from build123d import *

# Parameters (mm, degrees)
F0_R     = 3.302
F1_DEPTH = 6.35


with BuildPart() as f1:
    # F0 (on Top) → F1 (new body)
    with BuildSketch(Plane.XY):
        with BuildLine():
            ThreePointArc((12.671918, -0.844097), (12.692977, -0.422282), (12.7, 0))
            ThreePointArc((12.7, 0), (12.692977, 0.422282), (12.671918, 0.844097))
            ThreePointArc((12.671918, 0.844097), (12.507058, 2.205332), (12.196406, 3.540859))
            ThreePointArc((12.196406, 3.540859), (11.934096, 4.343656), (11.619009, 5.127243))
            ThreePointArc((11.619009, 5.127243), (10.998523, 6.35), (10.249828, 7.498736))
            ThreePointArc((10.249828, 7.498736), (9.728764, 8.163403), (9.164677, 8.791968))
            ThreePointArc((9.164677, 8.791968), (8.163403, 9.728764), (7.066969, 10.552154))
            ThreePointArc((7.066969, 10.552154), (6.35, 10.998523), (5.604949, 11.396251))
            ThreePointArc((5.604949, 11.396251), (4.343656, 11.934096), (3.031729, 12.332827))
            ThreePointArc((3.031729, 12.332827), (2.205332, 12.507058), (1.369182, 12.625979))
            ThreePointArc((1.369182, 12.625979), (0.685591, 12.681481), (0, 12.7))
            ThreePointArc((0, 12.7), (-0.685591, 12.681481), (-1.369182, 12.625979))
            ThreePointArc((-1.369182, 12.625979), (-2.205332, 12.507058), (-3.031729, 12.332827))
            ThreePointArc((-3.031729, 12.332827), (-4.343656, 11.934096), (-5.604949, 11.396251))
            ThreePointArc((-5.604949, 11.396251), (-6.35, 10.998523), (-7.066969, 10.552154))
            ThreePointArc((-7.066969, 10.552154), (-8.163403, 9.728764), (-9.164677, 8.791968))
            ThreePointArc((-9.164677, 8.791968), (-9.728764, 8.163403), (-10.249828, 7.498736))
            ThreePointArc((-10.249828, 7.498736), (-10.998523, 6.35), (-11.619009, 5.127243))
            ThreePointArc((-11.619009, 5.127243), (-11.934096, 4.343656), (-12.196406, 3.540859))
            ThreePointArc((-12.196406, 3.540859), (-12.507058, 2.205332), (-12.671918, 0.844097))
            ThreePointArc((-12.671918, 0.844097), (-12.7, 0), (-12.671918, -0.844097))
            ThreePointArc((-12.671918, -0.844097), (-12.507058, -2.205332), (-12.196406, -3.540859))
            ThreePointArc((-12.196406, -3.540859), (-11.934096, -4.343656), (-11.619009, -5.127243))
            ThreePointArc((-11.619009, -5.127243), (-10.998523, -6.35), (-10.249828, -7.498736))
            ThreePointArc((-10.249828, -7.498736), (-9.728764, -8.163403), (-9.164677, -8.791968))
            ThreePointArc((-9.164677, -8.791968), (-8.163403, -9.728764), (-7.066969, -10.552154))
            ThreePointArc((-7.066969, -10.552154), (-6.35, -10.998523), (-5.604949, -11.396251))
            ThreePointArc((-5.604949, -11.396251), (-4.343656, -11.934096), (-3.031729, -12.332827))
            ThreePointArc((-3.031729, -12.332827), (-2.205332, -12.507058), (-1.369182, -12.625979))
            ThreePointArc((-1.369182, -12.625979), (0, -12.7), (1.369182, -12.625979))
            ThreePointArc((1.369182, -12.625979), (2.205332, -12.507058), (3.031729, -12.332827))
            ThreePointArc((3.031729, -12.332827), (4.343656, -11.934096), (5.604949, -11.396251))
            ThreePointArc((5.604949, -11.396251), (6.35, -10.998523), (7.066969, -10.552154))
            ThreePointArc((7.066969, -10.552154), (8.163403, -9.728764), (9.164677, -8.791968))
            ThreePointArc((9.164677, -8.791968), (9.728764, -8.163403), (10.249828, -7.498736))
            ThreePointArc((10.249828, -7.498736), (10.998523, -6.35), (11.619009, -5.127243))
            ThreePointArc((11.619009, -5.127243), (11.934096, -4.343656), (12.196406, -3.540859))
            ThreePointArc((12.196406, -3.540859), (12.507058, -2.205332), (12.671918, -0.844097))
        make_face()
        Circle(F0_R, mode=Mode.SUBTRACT)
        with BuildLine():
            ThreePointArc((12.196406, 3.540859), (12.507058, 2.205332), (12.671918, 0.844097))
            Line((12.671918, 0.844097), (14.570677, 2.569203))
            Line((14.570677, 2.569203), (12.196406, 3.540859))
        make_face()
        with BuildLine():
            Line((14.570677, -2.569203), (12.671918, -0.844097))
            ThreePointArc((12.671918, -0.844097), (12.507058, -2.205332), (12.196406, -3.540859))
            Line((12.196406, -3.540859), (14.570677, -2.569203))
        make_face()
        with BuildLine():
            ThreePointArc((10.249828, 7.498736), (10.998523, 6.35), (11.619009, 5.127243))
            Line((11.619009, 5.127243), (12.813238, 7.397727))
            Line((12.813238, 7.397727), (10.249828, 7.498736))
        make_face()
        with BuildLine():
            Line((12.813238, -7.397727), (11.619009, -5.127243))
            ThreePointArc((11.619009, -5.127243), (10.998523, -6.35), (10.249828, -7.498736))
            Line((10.249828, -7.498736), (12.813238, -7.397727))
        make_face()
        with BuildLine():
            ThreePointArc((7.066969, 10.552154), (8.163403, 9.728764), (9.164677, 8.791968))
            Line((9.164677, 8.791968), (9.510334, 11.333975))
            Line((9.510334, 11.333975), (7.066969, 10.552154))
        make_face()
        with BuildLine():
            Line((9.510334, -11.333975), (9.164677, -8.791968))
            ThreePointArc((9.164677, -8.791968), (8.163403, -9.728764), (7.066969, -10.552154))
            Line((7.066969, -10.552154), (9.510334, -11.333975))
        make_face()
        with BuildLine():
            ThreePointArc((3.031729, 12.332827), (4.343656, 11.934096), (5.604949, 11.396251))
            Line((5.604949, 11.396251), (5.060343, 13.903178))
            Line((5.060343, 13.903178), (3.031729, 12.332827))
        make_face()
        with BuildLine():
            Line((5.060343, -13.903178), (5.604949, -11.396251))
            ThreePointArc((5.604949, -11.396251), (4.343656, -11.934096), (3.031729, -12.332827))
            Line((3.031729, -12.332827), (5.060343, -13.903178))
        make_face()
        with BuildLine():
            ThreePointArc((0, 12.7), (0.685591, 12.681481), (1.369182, 12.625979))
            Line((1.369182, 12.625979), (0, 14.795453))
            Line((0, 14.795453), (0, 12.7))
        make_face()
        with BuildLine():
            Line((0, -14.795453), (1.369182, -12.625979))
            ThreePointArc((1.369182, -12.625979), (0, -12.7), (-1.369182, -12.625979))
            Line((-1.369182, -12.625979), (0, -14.795453))
        make_face()
        with BuildLine():
            ThreePointArc((-1.369182, 12.625979), (-0.685591, 12.681481), (0, 12.7))
            Line((0, 12.7), (0, 14.795453))
            Line((0, 14.795453), (-1.369182, 12.625979))
        make_face()
        with BuildLine():
            Line((-5.060343, -13.903178), (-3.031729, -12.332827))
            ThreePointArc((-3.031729, -12.332827), (-4.343656, -11.934096), (-5.604949, -11.396251))
            Line((-5.604949, -11.396251), (-5.060343, -13.903178))
        make_face()
        with BuildLine():
            ThreePointArc((-5.604949, 11.396251), (-4.343656, 11.934096), (-3.031729, 12.332827))
            Line((-3.031729, 12.332827), (-5.060343, 13.903178))
            Line((-5.060343, 13.903178), (-5.604949, 11.396251))
        make_face()
        with BuildLine():
            Line((-9.510334, -11.333975), (-7.066969, -10.552154))
            ThreePointArc((-7.066969, -10.552154), (-8.163403, -9.728764), (-9.164677, -8.791968))
            Line((-9.164677, -8.791968), (-9.510334, -11.333975))
        make_face()
        with BuildLine():
            ThreePointArc((-9.164677, 8.791968), (-8.163403, 9.728764), (-7.066969, 10.552154))
            Line((-7.066969, 10.552154), (-9.510334, 11.333975))
            Line((-9.510334, 11.333975), (-9.164677, 8.791968))
        make_face()
        with BuildLine():
            Line((-12.813238, -7.397727), (-10.249828, -7.498736))
            ThreePointArc((-10.249828, -7.498736), (-10.998523, -6.35), (-11.619009, -5.127243))
            Line((-11.619009, -5.127243), (-12.813238, -7.397727))
        make_face()
        with BuildLine():
            ThreePointArc((-11.619009, 5.127243), (-10.998523, 6.35), (-10.249828, 7.498736))
            Line((-10.249828, 7.498736), (-12.813238, 7.397727))
            Line((-12.813238, 7.397727), (-11.619009, 5.127243))
        make_face()
        with BuildLine():
            Line((-14.570677, -2.569203), (-12.196406, -3.540859))
            ThreePointArc((-12.196406, -3.540859), (-12.507058, -2.205332), (-12.671918, -0.844097))
            Line((-12.671918, -0.844097), (-14.570677, -2.569203))
        make_face()
        with BuildLine():
            ThreePointArc((-12.671918, 0.844097), (-12.507058, 2.205332), (-12.196406, 3.540859))
            Line((-12.196406, 3.540859), (-14.570677, 2.569203))
            Line((-14.570677, 2.569203), (-12.671918, 0.844097))
        make_face()
    extrude(amount=F1_DEPTH)


solid = f1.part
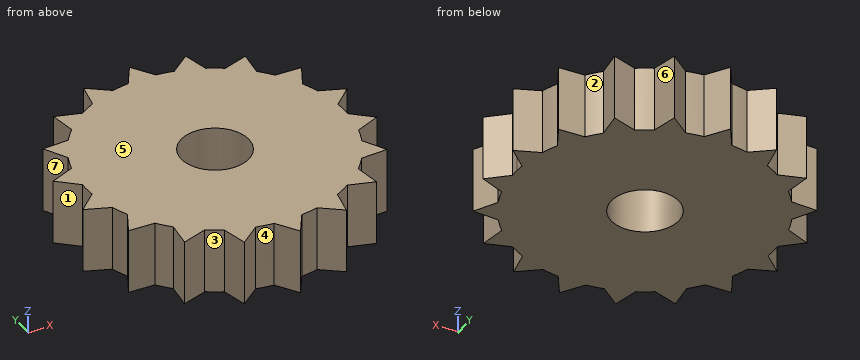
CAD build for the part. Positions are in the model's coordinates, mm. Face numbers are marked on the shaded views. A direction names the side the tool comes from. Give positions to 0.01 mm unless a question says otherwise; leave off trailing zeros. Write each loop counter-clockwise with the first axis right and the second up, starting at its lowest first coordinate (ties: lowest second). Pieces come first, ordered by that corner, then holes. Notation, with made-up numbers: (-36, -34) - (-24, -34) arc R6 ccw to (-24, -29) - close; hole circle Ø7 at (-35.5, 53). An arc over 180 degrees is marked (long way). Put each result on its own line as item: value.
(1) Drop flat-ended pins along their axis: pin 1 Ø1.5 at (y, z) = (-6.5, 3) entering from -X; pin 2 Ø2 at (y, z) = (-9.5, 1) entering from +X; pin 3 Ø2 at (y, z) = (5, 5) entering from -X. Give the stop position or say it passes through.
Working result:
pin 1: x = -12.74
pin 2: x = 9.44
pin 3: x = -12.08
(2) Pull direction X, two halves, no side cores. Call the marked faces 4, 5, 6 and 7: released by +X, released by -X, zero draft, split by the parting line, or undercut.
Working result:
face 4: undercut
face 5: zero draft
face 6: released by +X
face 7: released by -X
(3) Tool access for the marked faces 1, 2 and 3: list every direction of +Z, -Z, +X, -X, +Y, -Y with a clear straight run to the whole face (end or side of a thin tool).
Working result:
face 1: +Z, -Z, -X
face 2: +Z, -Z, +X
face 3: +Z, -Z, -Y
(4) Saw through at B-B (x = -11.25). List the corners of the cut face in (y, z), then the cut area to 3 significant figures.
Working result:
outline: (-7.46, 0) - (7.46, 0) - (7.46, 6.35) - (-7.46, 6.35) - close
area: 94.7 mm^2
(5) Wall check: L1, parallel to X at y = 1.25, z = 3; L2, parallel to Y at x = -1.25, z = 1.75; L3, parallel to X at y = -2.75, z = 4.5. Give the ranges that are in metal, low to high.
Working result:
L1: -13.12 to -3.06, 3.06 to 13.12
L2: -12.81 to -3.06, 3.06 to 12.81
L3: -14.13 to -1.83, 1.83 to 14.13
(6) Saw through at A-A (x = 1). List the corners of the cut face in (y, z).
Working result:
outline: (-13.21, 0) - (-3.15, 0) - (-3.15, 6.35) - (-13.21, 6.35) - close; (3.15, 0) - (13.21, 0) - (13.21, 6.35) - (3.15, 6.35) - close
